Autodesk Inventor part; units mm, degrees
ref_plane "YZ Plane" through (0, 0, 0) normal (1, 0, 0) x (0, 1, 0)
ref_plane "XZ Plane" through (0, 0, 0) normal (0, 1, 0) x (-1, 0, 0)
ref_plane "XY Plane" through (0, 0, 0) normal (0, 0, 1) x (1, 0, 0)
sketch "Sketch1" plane through (0, 0, 0) normal (0, 1, 0) x (-1, 0, 0)
  line L0 (-9.5, -12.625) -> (9.5, -12.625)
  line L1 (9.5, -12.625) -> (9.5, 12.625)
  line L2 (9.5, 12.625) -> (-9.5, 12.625)
  line L3 (-9.5, 12.625) -> (-9.5, -12.625)
  line L4 (-9.5, -12.625) -> (9.5, 12.625) construction
  line L5 (9.5, -12.625) -> (-9.5, 12.625) construction
  point P0 (0, 0)
  dimension "d0" = 19
  dimension "d1" = 25.25
extrude "Extrusion1" add sketch "Sketch1" along normal blind 10.75
shell "Shell1" thickness 1 removed faces 1 at (3.1667, 10.75, 4.2083)
sketch "Sketch2" plane through (9.5, 0, 12.625) normal (1, 0, 0) x (0, 0, -1)
  line L0 (1, 1) -> (24.25, 1)
  circle A0 centre (6.5, 7) radius 3.5
  line L1 (1, 1) -> (1, 10.75)
  line L2 (2, 3.75) -> (5.201, 3.75)
  line L3 (7.799, 3.75) -> (24, 3.75)
  point P0 (12.625, 0)
  dimension "d6" = 7
  dimension "d8" = 2
extrude "Extrusion2" cut sketch "Sketch2" against normal blind 10.75
sketch "Sketch3" plane through (0, 10.75, 0) normal (0, 1, 0) x (1, 0, 0)
  line L0 (-8.5, -11.625) -> (-8.5, 11.625)
  line L1 (-8.5, 11.625) -> (8.5, 11.625)
  line L2 (-9.5, -12.625) -> (9.5, -12.625)
  line L3 (9.5, -12.625) -> (9.5, 12.625)
  line L4 (9.5, 12.625) -> (-9.5, 12.625)
  line L5 (-9.5, 12.625) -> (-9.5, -12.625)
  line L6 (-9.5, -12.625) -> (9.5, -12.625)
  line L7 (9.5, -12.625) -> (9.5, 12.625)
  line L8 (9.5, 12.625) -> (-9.5, 12.625)
  line L9 (-9.5, 12.625) -> (-9.5, -12.625)
  line L10 (3.75, 6.875) -> (-3.75, 6.875)
  line L11 (-3.75, 6.875) -> (-3.75, -0.625)
  line L12 (-3.75, -0.625) -> (3.75, -0.625)
  line L13 (3.75, -0.625) -> (3.75, 6.875)
  line L14 (3.75, 6.875) -> (-3.75, -0.625) construction
  line L15 (-3.75, 6.875) -> (3.75, -0.625) construction
  point P0 (0, 0)
  point P1 (0, 3.125)
  dimension "d11" = 8.5
  dimension "d12" = 8.5
  dimension "d13" = 7.5
  dimension "d14" = 7.5
extrude "Extrusion3" add sketch "Sketch3" along normal blind 1
fillet "Fillet1" radius 1 4 edges at (9.5, 5.875, -12.625) (-9.5, 5.875, -12.625) (-9.5, 5.875, 12.625) (9.5, 5.875, 12.625)
properties part number "carcasaXeotype_BUTTON"
Model file for the job. Use its own axes, mm. A direction names the side the tool comes from. Give positions to 0.01 mm unless a question says otherwise; leave off trailing zeros. Write each loop counter-clockwise with the first axis right and the second up, starting at its lowest first coordinate (ties: lowest second). Pieces come first, ordered by that corner, then holes. Notation, with made-up numbers: M 47.5,-21.75 L 75.5,-21.75 A25 ccw 75.5,17.25 Z; hole C 8,-7.5 d10. An arc over 180 degrees is marked long. One line per item, written item: value. Start each with the question number.
Q1. Saw through at C-C, the plane y = 7. Write the cut outline in (x, z) (3 decimals).
Q2. Two-plate mould, pull along X, no slides. Class faces 1 (the flat face through (0, 6, 12.625)), 2 (the cylindrical face through (-9.215, 5.957, 12.324)), 3 (the flat face through (0, 6, -11.625)), 4 (the flat face through (0, 11, -6.875)): +X half, -X half, draft (parallel to the pull), parting line (faces both ways), or undercut.
Q3. 3-axis set-ups, long thin cutter, end or side, ignore diameter. For faces 5 (the flat face through (-3.75, 11, -3)), 6 (the cylindrical face through (9.007, 3.583, 6.884)), 7 (the cylindrical face through (-9.215, 5.793, -12.324)), 8 (the flat face through (0, 6, -12.625)), 9 (the flat face through (0, 10.75, 2)): which of +Z, -Z, +X, -X, +Y, -Y reach the whole face in a straight line?
Q4. Saw through at D-D, the plane y = 2. Write the cut outline in (x, z) (3 decimals).
Q5. Saw through at B-B, the plane x = 7.75. Write the cut outline in (y, z) (3 decimals), plus the area to 3 significant figures.
Q6. Probe probe 1 along X at (y, z) = (5.5, -2.75); probe 2 along Y at (x, z) = (4, -11.25); probe 3 along Z at (x, y) = (7.5, 8.5) (3 decimals). List the from-to ranges inside material, lowest first. Write a range as [from, to].
Q7. Saw through at A-A, the plane z = 1.5. Write the cut outline in (x, y), plus the area to 3 significant figures.
Output values:
1. outline: M -9.5,-11.625 A1 ccw -8.5,-12.625 L 8.5,-12.625 A1 ccw 9.5,-11.625 L 9.5,2.625 L 8.5,2.625 L 8.5,-11.625 L -8.5,-11.625 L -8.5,11.625 L 8.5,11.625 L 8.5,9.625 L 9.5,9.625 L 9.5,11.625 A1 ccw 8.5,12.625 L -8.5,12.625 A1 ccw -9.5,11.625 Z
2. face 1: draft
2. face 2: -X half
2. face 3: undercut
2. face 4: undercut
3. face 5: +Y
3. face 6: +X
3. face 7: -Z, -X, +Y, -Y
3. face 8: -Z, +X, -X, +Y, -Y
3. face 9: none
4. outline: M -9.5,-11.625 A1 ccw -8.5,-12.625 L 8.5,-12.625 A1 ccw 9.5,-11.625 L 9.5,11.625 A1 ccw 8.5,12.625 L -8.5,12.625 A1 ccw -9.5,11.625 Z; hole M -8.5,-11.625 L 8.5,-11.625 L 8.5,11.625 L -8.5,11.625 Z
5. outline: M 0,-12.625 L 11.75,-12.625 L 11.75,12.625 L 0,12.625 Z; hole M 1,-11.625 L 10.75,-11.625 L 10.75,11.625 L 1,11.625 Z
5. area: 70.0 mm²
6. probe 1: x = [-9.5, -8.5], [8.5, 9.5]
6. probe 2: y = [0, 1], [10.75, 11.75]
6. probe 3: z = [-12.625, -11.625], [11.625, 12.625]
7. outline: M -9.5,0 L 9.5,0 L 9.5,11.75 L -9.5,11.75 Z; hole M -8.5,1 L 8.5,1 L 8.5,10.75 L -8.5,10.75 Z
7. area: 57.5 mm²
